Geometry check sheet. Reference: the model listing, model coordinates, mm. A direction names the side the tool comes from. Round coordinates to 2 decimals unless told otherwise and drop trailing zeros. Loops run counter-clockwise (first coordinate to the right, second up) from the corner with the lowest first, then second, coordinate; pieces in that order, holes last.
```python
from build123d import *

# Parameters (mm, degrees)
SKETCH2_W                   = 72.968
SKETCH2_H                   = 24.996
BASE_FLANGE1_DEPTH          = 1.016
EDGE_FLANGE1_DEPTH          = 21.948
FILLET1_R                   = 2
TAP_DRILL_FOR_M3X0_5_TAP1_D = 2.5


# Sheet-metal steps are written as plain solids
with BuildPart() as part:
    # Sketch2 → Base-Flange1 (new body)
    with BuildSketch(Plane.XY):
        with Locations((-36.484, -12.498)):
            Rectangle(SKETCH2_W, SKETCH2_H)
    extrude(amount=-BASE_FLANGE1_DEPTH)

    # Edge-Flange1 section (across the edge) → Edge-Flange1 (add)
    with BuildSketch(Plane(origin=(-73.984, -24.996, -1.016), x_dir=(1, 0, 0), z_dir=(0, 1, 0))):
        with BuildLine():
            Line((-1.016, 1.016), (-1.016, 8))
            Line((-1.016, 8), (0, 8))
            Line((0, 8), (0, 1.016))
            ThreePointArc((0, 1.016), (0.29757951, 0.29757951), (1.016, 0))
            Line((1.016, 0), (1.016, -1.016))
            ThreePointArc((1.016, -1.016), (-0.420840979, -0.420840979), (-1.016, 1.016))
        make_face()
    extrude(amount=EDGE_FLANGE1_DEPTH)

    # Fillet1
    fillet1_edges = [part.edges().sort_by_distance(p)[0] for p in [
        (-74.492, -24.996, -9.016),
        (-74.492, -3.048, -9.016),
        (-72.968, 0, -0.508),
    ]]
    fillet(fillet1_edges, radius=FILLET1_R)

    # Tap Drill for M3x0.5 Tap1 (through all)
    with Locations(Plane.ZY.offset(75)):
        with Locations((-5.524, -6.048)):
            Hole(TAP_DRILL_FOR_M3X0_5_TAP1_D / 2)

    # Mirror1: part across plane


with BuildPart() as part_1:
    add(part.part)
    add(part.part.mirror(Plane(origin=(0, -24.996, -1.016), x_dir=(0, 0, 1), z_dir=(1, 0, 0))))


solid = part_1.part
```
1) Gauge pin test, flat ends, axial feed: pin 1 (1 mm diameter, centred on x = -74, z = -4, fed in from +Y); pin 2 (1 mm diameter, centred on x = -12, y = -21, fed in from -Z); pin 3 (0.5 mm diameter, centred on y = -2.5, z = -0.5, fed in from +X). Record the tip position at first contact, or that the pin passes through.
Report:
pin 1: stops at y = -3.05
pin 2: stops at z = -1.02
pin 3: stops at x = 72.97
2) Sectioned sample at C-C, the plane x = -15.5. Record the cut outline in (y, z).
Report:
outline: (-25, -1.02) - (0, -1.02) - (0, 0) - (-25, 0) - close
3) Sectioned sample at A-A, the plane y = -15.5. Record the cut outline in (x, z).
Report:
outline: (-75, -9.02) - (-73.98, -9.02) - (-73.98, -2.03) arc R1.02 cw to (-72.97, -1.02) - (72.97, -1.02) arc R1.02 cw to (73.98, -2.03) - (73.98, -9.02) - (75, -9.02) - (75, -2.03) arc R2.03 ccw to (72.97, 0) - (-72.97, 0) arc R2.03 ccw to (-75, -2.03) - close
4) Sectioned sample at B-B, the plane z = -5.5. Record the cut outline in (x, y).
Report:
outline: (-75, -25) - (-73.98, -25) - (-73.98, -7.3) - (-75, -7.3) - close; (-75, -4.8) - (-73.98, -4.8) - (-73.98, -3.05) - (-75, -3.05) - close; (73.98, -25) - (75, -25) - (75, -7.3) - (73.98, -7.3) - close; (73.98, -4.8) - (75, -4.8) - (75, -3.05) - (73.98, -3.05) - close
5) Scan lines: line 1 along X through (y, z) = (-5.75, -2); line 2 along Z through (x, y) = (1, -7.75); line 3 along X through (y, z) = (-11, -0.75). Record each from-to range of solid material in increasing order.
Report:
line 1: x = -75 to -73.98, 73.98 to 75
line 2: z = -1.02 to 0
line 3: x = -74.54 to 74.54
6) Access from +Z, -Z, +X, -X, +Y, -Y to the whole of each face (thin tool, end or side, straight path). Record for faces 5 (the face through (-75, -14, -5)), 6 (the face through (1, -12, -1.016)).
Report:
face 5: +Z, -Z, -X, +Y, -Y
face 6: -Z, +Y, -Y
7) Mould release check, pull along Y, two halves, no side actions. Record for faces 1 (the face through (-0.4, -24.996, -0.7)), 2 (the face through (1, -12, 0)), 3 (the face through (74.485, -7.268, -5.253)), 4 (the face through (-74.485, -7.268, -5.253)): +Y half, -Y half, draft (parallel to the pull), parting line (faces both ways), or undercut.
Report:
face 1: -Y half
face 2: draft
face 3: undercut
face 4: undercut
